Read the model definition and answer for the solid it produces. Units are mm, in the model's axes. Give positions to 0.01 mm unless a question says otherwise; leave off trailing zeros. Write each loop counter-clockwise with the first axis right and the second up, starting at its lowest first coordinate (ties: lowest second). Pieces come first, ordered by that corner, then holes.
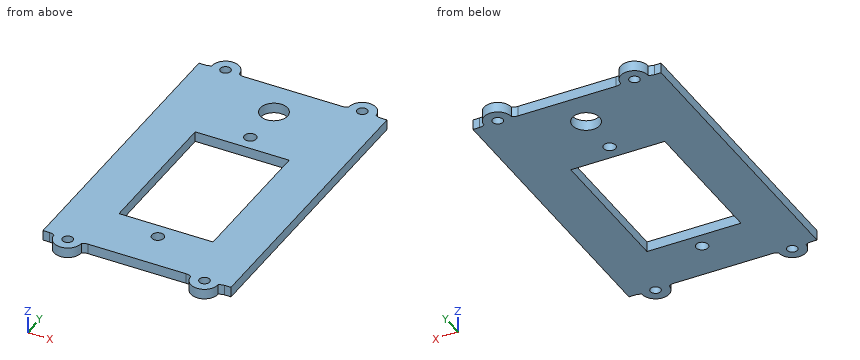
```python
from build123d import *

# Parameters (mm, degrees)
SKETCH1_R           = 1.5
BOSS_EXTRUDE1_DEPTH = 3
SKETCH2_R           = 4
SKETCH2_R_2         = 1.75
SKETCH2_W           = 27.5
SKETCH2_H           = 42
CUT_EXTRUDE1_DEPTH  = 55.968172609


with BuildPart() as part:
    # Sketch1 → Boss-Extrude1 (new body)
    with BuildSketch(Plane.XY):
        with BuildLine():
            ThreePointArc((-14.341687605, -43), (-15.207713009, -43.127718677), (-16, -43.5))
            ThreePointArc((-16, -43.5), (-20, -47.5), (-24, -43.5))
            ThreePointArc((-24, -43.5), (-24.792286991, -43.127718677), (-25.658312395, -43))
            Line((-25.658312395, -43), (-27.5, -43))
            Line((-27.5, -43), (-27.5, 43))
            Line((-27.5, 43), (-25.658312395, 43))
            ThreePointArc((-25.658312395, 43), (-24.792286991, 43.127718677), (-24, 43.5))
            ThreePointArc((-24, 43.5), (-20, 47.5), (-16, 43.5))
            ThreePointArc((-16, 43.5), (-15.207713009, 43.127718677), (-14.341687605, 43))
            Line((-14.341687605, 43), (-10.658312395, 43))
            Line((-10.658312395, 43), (10.658312395, 43))
            Line((10.658312395, 43), (14.341687605, 43))
            ThreePointArc((14.341687605, 43), (15.207713009, 43.127718677), (16, 43.5))
            ThreePointArc((16, 43.5), (20, 47.5), (24, 43.5))
            ThreePointArc((24, 43.5), (24.792286991, 43.127718677), (25.658312395, 43))
            Line((25.658312395, 43), (27.5, 43))
            Line((27.5, 43), (27.5, -43))
            Line((27.5, -43), (25.658312395, -43))
            ThreePointArc((25.658312395, -43), (24.792286991, -43.127718677), (24, -43.5))
            ThreePointArc((24, -43.5), (20, -47.5), (16, -43.5))
            ThreePointArc((16, -43.5), (15.207713009, -43.127718677), (14.341687605, -43))
            Line((14.341687605, -43), (10.658312395, -43))
            Line((10.658312395, -43), (-10.658312395, -43))
            Line((-10.658312395, -43), (-14.341687605, -43))
        make_face()
        with Locations((20, -43.5)):
            Circle(SKETCH1_R, mode=Mode.SUBTRACT)
        with Locations((-20, -43.5)):
            Circle(SKETCH1_R, mode=Mode.SUBTRACT)
        with Locations((20, 43.5)):
            Circle(SKETCH1_R, mode=Mode.SUBTRACT)
        with Locations((-20, 43.5)):
            Circle(SKETCH1_R, mode=Mode.SUBTRACT)
    extrude(amount=BOSS_EXTRUDE1_DEPTH)

    # Sketch2 → Cut-Extrude1 (cut, through all)
    with BuildSketch(Plane.XY):
        with Locations((0, 32.5)):
            Circle(SKETCH2_R)
        with Locations((0, 19.5)):
            Circle(SKETCH2_R_2)
        with Locations((0, -31.5)):
            Circle(SKETCH2_R_2)
        with Locations((0, -6)):
            Rectangle(SKETCH2_W, SKETCH2_H)
    extrude(amount=CUT_EXTRUDE1_DEPTH, mode=Mode.SUBTRACT)


solid = part.part
```
Item 1: Find the intervals of material crossed by line 1 along Y through (x, z) = (0, 0.9); line 2 along Y through (x, z) = (20, 1.75); line 3 along X through (y, z) = (32.5, 1.1), in increasing order.
Result set:
line 1: y = -43 to -33.25, -29.75 to -27, 15 to 17.75, 21.25 to 28.5, 36.5 to 43
line 2: y = -47.5 to -45, -42 to 42, 45 to 47.5
line 3: x = -27.5 to -4, 4 to 27.5
Item 2: Section A-A (x = -20) is taken. Write down the section's boundary in (y, z), and give its area (3 significant figures).
Result set:
outline: (-47.5, 0) - (-45, 0) - (-45, 3) - (-47.5, 3) - close; (-42, 0) - (42, 0) - (42, 3) - (-42, 3) - close; (45, 0) - (47.5, 0) - (47.5, 3) - (45, 3) - close
area: 267 mm2
Item 3: Each of these flat-tipped pins is pushed along its axis until it touches: pin 1 Ø0.6 at (x, z) = (26.5, 2) entering from -Y; pin 2 Ø0.6 at (x, z) = (-26.5, 1) entering from +Y; pin 3 Ø1 at (x, z) = (-18.5, 2.5) entering from -Y. Where does it stop, or does it pass through?
Result set:
pin 1: stops at y = -43
pin 2: stops at y = 43
pin 3: stops at y = -47.37
Item 4: Section D-D (x = -7.5) is taken. Write down the section's boundary in (y, z), and give its area (3 significant figures).
Result set:
outline: (-43, 0) - (-27, 0) - (-27, 3) - (-43, 3) - close; (15, 0) - (43, 0) - (43, 3) - (15, 3) - close
area: 132 mm2
Item 5: Section C-C (y = 14) is taken. Write down the section's boundary in (x, z), and give its area (3 significant figures).
Result set:
outline: (-27.5, 0) - (-13.75, 0) - (-13.75, 3) - (-27.5, 3) - close; (13.75, 0) - (27.5, 0) - (27.5, 3) - (13.75, 3) - close
area: 82.5 mm2
Item 6: Section B-B (z = 0.8) is taken. Give the number of separate pieces and of enclosed holes in the cut face, and give its area (3 significant figures).
Result set:
separate pieces: 1
enclosed holes: 8
area: 3,600 mm2
